```python
from build123d import *

# Parameters (mm, degrees)
F0_R     = 9.525
F1_DEPTH = 25.4
F3_DEPTH = 25.4
F4_DEPTH = 11.0998
F6_DEPTH = 2.54


with BuildPart() as f1:
    # F0 (on Front) → F1 (new body)
    with BuildSketch(Plane.XZ):
        Circle(F0_R)
    extrude(amount=F1_DEPTH)

    # F2 (on Front) → F3 (cut)
    with BuildSketch(Plane.XZ):
        with BuildLine():
            ThreePointArc((-4.7625, 0), (-3.367596, -3.367596), (0, -4.7625))
            ThreePointArc((0, -4.7625), (3.367596, -3.367596), (4.7625, 0))
            ThreePointArc((4.7625, 0), (3.367596, 3.367596), (0, 4.7625))
            ThreePointArc((0, 4.7625), (-3.367596, 3.367596), (-4.7625, 0))
        make_face()
    extrude(amount=F3_DEPTH, mode=Mode.SUBTRACT)

    # F2 (on Front) → F4 (cut)
    with BuildSketch(Plane.XZ):
        with BuildLine():
            Line((-4.7625, 0), (-4.7625, -4.7625))
            Line((-4.7625, -4.7625), (0, -4.7625))
            ThreePointArc((0, -4.7625), (-3.367596, -3.367596), (-4.7625, 0))
        make_face()
        with BuildLine():
            ThreePointArc((4.7625, 0), (3.367596, -3.367596), (0, -4.7625))
            Line((0, -4.7625), (4.7625, -4.7625))
            Line((4.7625, -4.7625), (4.7625, 0))
        make_face()
        with BuildLine():
            Line((-4.7625, 4.7625), (-4.7625, 0))
            ThreePointArc((-4.7625, 0), (-3.367596, 3.367596), (0, 4.7625))
            Line((0, 4.7625), (-4.7625, 4.7625))
        make_face()
        with BuildLine():
            ThreePointArc((0, 4.7625), (3.367596, 3.367596), (4.7625, 0))
            Line((4.7625, 0), (4.7625, 4.7625))
            Line((4.7625, 4.7625), (0, 4.7625))
        make_face()
    extrude(amount=F4_DEPTH, mode=Mode.SUBTRACT)

    # F5 (on face) → F6 (cut)
    with BuildSketch(Plane.XZ.offset(25.4)):
        Polygon((7.3025, 0), (3.65125, 6.324151), (-3.65125, 6.324151), (-7.3025, 0), (-3.65125, -6.324151), (3.65125, -6.324151), align=None)
    extrude(amount=-F6_DEPTH, mode=Mode.SUBTRACT)


solid = f1.part
```
Can you work these out from the model? Positions are in its coordinate system, mm. A direction names the side the tool comes from. Give positions to 0.01 mm unless a question says otherwise; leave off trailing zeros. Write each loop counter-clockwise with the first axis right and the second up, starting at its lowest first coordinate (ties: lowest second). Pieces come first, ordered by that corner, then holes. Notation, with made-up numbers: (56.25, -4) -> (64.25, -4) arc R28 cw to (64.25, 33) -> close; hole circle Ø9 at (-5, -23.75). An arc over 180 degrees is marked (long way). One line per item, written item: value.
Q1. Imagine slicing it at B-B on z = 0.75. Please give me the cut outline in (x, y), and give its area (3 significant figures).
Results found:
outline: (-9.5, -25.4) -> (-6.87, -25.4) -> (-6.87, -22.86) -> (-4.7, -22.86) -> (-4.7, -11.1) -> (-4.76, -11.1) -> (-4.76, 0) -> (-9.5, 0) -> close; (4.7, -22.86) -> (6.87, -22.86) -> (6.87, -25.4) -> (9.5, -25.4) -> (9.5, 0) -> (4.76, 0) -> (4.76, -11.1) -> (4.7, -11.1) -> close
area: 231 mm^2
Q2. We'd pull the mould along X, two halves only. Please class faces 1 (the face through (6.2, -25.4, 2.3)), 2 (the face through (0, -5, 4.762)), 3 (the face through (-7.559, -12.522, -5.796)): +X half, -X half, draft (parallel to the pull), parting line (faces both ways), or undercut.
Results found:
face 1: draft
face 2: undercut
face 3: parting line
Q3. Imagine slicing it at C-C on x = 3. Please give me the cut outline in (y, z), and give its area (3 significant figures).
Results found:
outline: (-25.4, -9.04) -> (0, -9.04) -> (0, -4.76) -> (-11.1, -4.76) -> (-11.1, -3.7) -> (-22.86, -3.7) -> (-22.86, -6.32) -> (-25.4, -6.32) -> close; (-25.4, 6.32) -> (-22.86, 6.32) -> (-22.86, 3.7) -> (-11.1, 3.7) -> (-11.1, 4.76) -> (0, 4.76) -> (0, 9.04) -> (-25.4, 9.04) -> close
area: 234 mm^2
Q4. For P1, Ø10, axis at x = 0.5, z = -0.5, coming from the -Y side; P2, Ø4, axis at x = -2.5, z = 1, coming from the +Y side; P3, Ø1, axis at x = -7.5, y = -17.5, coming from the -Z side; P4, Ø1.5, axis at y = -4.5, z = -3, coming from the +X side, each with a flat end and sliding along its axis, tell me the tip position at first contact or that it passes through.
Results found:
P1: stops at y = -22.86
P2: passes through
P3: stops at z = -6.46
P4: stops at x = 9.26
Q5. Please list where these lines run through material, in increasing order: line 1 (Z direction, x = 0.25, y = -13.5); line 2 (Z direction, x = -2, y = -2); line 3 (X direction, y = -10.75, z = -1.25). Write a range as [from, to].
Results found:
line 1: z = [-9.52, -4.76], [4.76, 9.52]
line 2: z = [-9.31, -4.76], [4.76, 9.31]
line 3: x = [-9.44, -4.76], [4.76, 9.44]
Q6. Which directions (+Z, -Z, +X, -X, +Y, -Y) give clear straight access to the entire face, cutting with the end or side of a thin tool? Please do faces 4 (the face through (0, -24, 6.324)), 5 (the face through (-4, -11.1, -4)), 6 (the face through (0, 0, -6)).
Results found:
face 4: -Y
face 5: +Y
face 6: +Z, -Z, +X, -X, +Y
